```python
from build123d import *
from build123d.topology import SkipClean

# Parameters (mm, degrees)
SKETCH1_R               = 101.6
BOSS_EXTRUDE1_DEPTH     = 12.7
BOSS_EXTRUDE3_DEPTH     = 177.8
FILLET3_R               = 43.18
SKETCH3_R               = 25.4
CUT_EXTRUDE1_DEPTH      = 229.600000167
CUT_EXTRUDE2_DEPTH      = 276.632670899
CUT_EXTRUDE2_DEPTH_BACK = 276.632670899
SKETCH4_R               = 14.2875
CUT_EXTRUDE3_DEPTH      = 276.6326709
CUT_EXTRUDE3_DEPTH_BACK = 276.6326709
FILLET4_R               = 22.86
SKETCH7_W               = 43.18
SKETCH7_H               = 10
BOSS_EXTRUDE4_DEPTH     = 42.418
BOSS_EXTRUDE5_DEPTH     = 43.18
FILLET5_R               = 17.78


with BuildPart() as part:
    # Sketch1 → Boss-Extrude1 (new body)
    with BuildSketch(Plane(origin=(0, 0, 0), x_dir=(1, 0, 0), z_dir=(0, 1, 0))):
        with Locations(Location((0, 0, 0), (0, 0, 270))):
            Circle(SKETCH1_R)
    extrude(amount=BOSS_EXTRUDE1_DEPTH)

    # Sketch2 → Boss-Extrude3 (add)
    with SkipClean():  # the faces are left unmerged after this step: merging them gives an invalid solid
        with BuildSketch(Plane(origin=(0, 12.7, 0), x_dir=(1, 0, 0), z_dir=(0, 1, 0))):
            with BuildLine():
                Line((-69.749231612, -34.987681034), (-95.385649738, -34.987681034))
                ThreePointArc((-95.385649738, -34.987681034), (-101.6, 0), (-95.385649738, 34.987681034))
                Line((-95.385649738, 34.987681034), (-69.749231612, 34.987681034))
                Line((-69.749231612, 34.987681034), (-69.749231612, -34.987681034))
            make_face()
            with BuildLine():
                Line((69.749231612, 34.987681034), (95.385649738, 34.987681034))
                ThreePointArc((95.385649738, 34.987681034), (101.6, 0), (95.385649738, -34.987681034))
                Line((95.385649738, -34.987681034), (69.749231612, -34.987681034))
                Line((69.749231612, -34.987681034), (69.749231612, 34.987681034))
            make_face()
        extrude(amount=BOSS_EXTRUDE3_DEPTH)

    # Fillet3
    # the kernel refuses this fillet: 43.18 mm, written as the material it adds along each edge
    with BuildSketch(Plane(origin=(-203.335649738, 12.7, -34.987681034), x_dir=(0, 0, -1), z_dir=(1, 0, 0))) as fillet3_piece_1_section:
        with BuildLine():
            CenterArc((FILLET3_R, FILLET3_R), FILLET3_R, 180, 90)
            Line((0, FILLET3_R), (0, 0))
            Line((0, 0), (FILLET3_R, 0))
        make_face()
    fillet3_piece_1 = extrude(amount=133.586418126, mode=Mode.PRIVATE)
    fillet3_piece_1 = fillet3_piece_1 & Plane(origin=(0, 23.799745308, 0), x_dir=(0, 0, 1), z_dir=(0, -1, 0)) * Cylinder(101.6, 440, mode=Mode.PRIVATE)
    add(fillet3_piece_1)
    with BuildSketch(Plane(origin=(203.335649738, 12.7, 34.987681034), x_dir=(0, 0, 1), z_dir=(-1, 0, 0))) as fillet3_piece_2_section:
        with BuildLine():
            CenterArc((FILLET3_R, FILLET3_R), FILLET3_R, 180, 90)
            Line((0, FILLET3_R), (0, 0))
            Line((0, 0), (FILLET3_R, 0))
        make_face()
    fillet3_piece_2 = extrude(amount=133.586418126, mode=Mode.PRIVATE)
    fillet3_piece_2 = fillet3_piece_2 & Plane(origin=(0, 23.799745308, 0), x_dir=(0, 0, 1), z_dir=(0, -1, 0)) * Cylinder(101.6, 440, mode=Mode.PRIVATE)
    add(fillet3_piece_2)
    with BuildSketch(Plane(origin=(69.749231612, 12.7, -34.987681034), x_dir=(0, 0, -1), z_dir=(1, 0, 0))) as fillet3_piece_3_section:
        with BuildLine():
            CenterArc((FILLET3_R, FILLET3_R), FILLET3_R, 180, 90)
            Line((0, FILLET3_R), (0, 0))
            Line((0, 0), (FILLET3_R, 0))
        make_face()
    fillet3_piece_3 = extrude(amount=133.586418126, mode=Mode.PRIVATE)
    fillet3_piece_3 = fillet3_piece_3 & Plane(origin=(0, 23.79973444, 0), x_dir=(0, 0, 1), z_dir=(0, -1, 0)) * Cylinder(101.6, 440, mode=Mode.PRIVATE)
    add(fillet3_piece_3)
    with BuildSketch(Plane(origin=(-69.749231612, 12.7, 34.987681034), x_dir=(0, 0, 1), z_dir=(-1, 0, 0))) as fillet3_piece_4_section:
        with BuildLine():
            CenterArc((FILLET3_R, FILLET3_R), FILLET3_R, 180, 90)
            Line((0, FILLET3_R), (0, 0))
            Line((0, 0), (FILLET3_R, 0))
        make_face()
    fillet3_piece_4 = extrude(amount=133.586418126, mode=Mode.PRIVATE)
    fillet3_piece_4 = fillet3_piece_4 & Plane(origin=(0, 23.79973444, 0), x_dir=(0, 0, 1), z_dir=(0, -1, 0)) * Cylinder(101.6, 440, mode=Mode.PRIVATE)
    add(fillet3_piece_4)

    # Sketch3 → Cut-Extrude1 (cut, through all)
    with BuildSketch(Plane(origin=(0, 12.7, 0), x_dir=(1, 0, 0), z_dir=(0, 1, 0))):
        with Locations(Location((0, 0, 0), (0, 0, 270))):
            Circle(SKETCH3_R)
    extrude(amount=-CUT_EXTRUDE1_DEPTH, mode=Mode.SUBTRACT)

    # Sketch4 → Cut-Extrude2 (cut, two sides: drawn at the far end of the back side and taken through both)
    with BuildSketch(Plane.ZY.offset(-69.749231612).offset(-CUT_EXTRUDE2_DEPTH_BACK)):
        with Locations((0, 165.1)):
            Circle(SKETCH4_R)
    extrude(amount=CUT_EXTRUDE2_DEPTH + CUT_EXTRUDE2_DEPTH_BACK, mode=Mode.SUBTRACT)

    # Sketch5 → Cut-Extrude3 (cut, two sides: drawn at the far end of the back side and taken through both)
    with BuildSketch(Plane.ZY.offset(-69.749231612).offset(-CUT_EXTRUDE3_DEPTH_BACK)):
        with BuildLine():
            Line((34.987681034, 160.366849855), (34.987681034, 209.992755937))
            Line((34.987681034, 209.992755937), (-34.987681034, 209.992755937))
            Line((-34.987681034, 209.992755937), (-34.987681034, 160.366849855))
            ThreePointArc((-34.987681034, 160.366849855), (0, 195.354530889), (34.987681034, 160.366849855))
        make_face()
    extrude(amount=CUT_EXTRUDE3_DEPTH + CUT_EXTRUDE3_DEPTH_BACK, mode=Mode.SUBTRACT)

    # Fillet4
    fillet4_edges = [part.edges().sort_by_distance(p)[0] for p in [
        (-84.890685507, 190.5, -17.780075547),
        (-84.890685507, 190.5, 17.780075547),
        (84.890685507, 190.5, -17.780075547),
        (84.890685507, 190.5, 17.780075547),
    ]]
    fillet(fillet4_edges, radius=FILLET4_R)

    # Sketch7 → Boss-Extrude4 (add)
    with BuildSketch(Plane(origin=(0, 12.7, 0), x_dir=(1, 0, 0), z_dir=(0, 1, 0))):
        with Locations((-48.159231612, 26.209)):
            Rectangle(SKETCH7_W, SKETCH7_H)
        with Locations((-48.159231612, -26.209)):
            Rectangle(SKETCH7_W, SKETCH7_H)
    extrude(amount=BOSS_EXTRUDE4_DEPTH)

    # Sketch8 → Boss-Extrude5 (add)
    with BuildSketch(Plane(origin=(-69.749231612, 0, 0), x_dir=(0, 0, -1), z_dir=(1, 0, 0))):
        Polygon((-21.209, 17.78), (-21.209, 12.7), (-16.891, 12.7), align=None)
        Polygon((16.891, 12.7), (21.209, 17.78), (21.209, 12.7), align=None)
    extrude(amount=BOSS_EXTRUDE5_DEPTH)

    # Fillet5
    fillet5_edges = [part.edges().sort_by_distance(p)[0] for p in [
        (-48.159231612, 12.7, -31.209),
        (-48.159231612, 12.7, 31.209),
    ]]
    fillet(fillet5_edges, radius=FILLET5_R)


solid = part.part
```
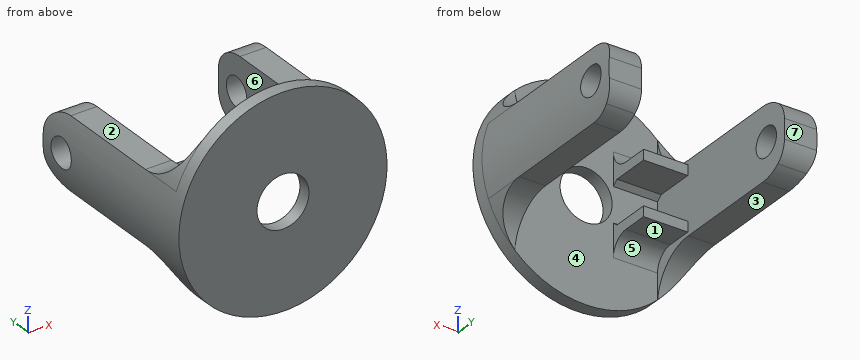
Build history of the part. All positions in model axes, mm. Face numbers are marked on the shaded views. A direction names the side the tool comes from. Round coordinates to 2 decimals unless told otherwise and drop trailing zeros. Loops run counter-clockwise (first coordinate to the right, second up) from the corner with the lowest first, then second, coordinate; pieces in that order, holes last.
Item 1: Saw through at C-C (y = 165.1). List the corners of the cut face in (x, z), then the cut area to 3 significant figures.
Item 2: Saw through at B-B (z = 0). List the corners of the cut face in (x, y).
Item 3: Saw through at A-A (x = 0). List the corners of the cut face in (y, z), then the cut area to 3 significant figures.
Item 4: Pin check, flat tips, straight feed: P1, Ø8, axis at x = 75, z = 29, coming from the +Y side; P2, Ø6, axis at y = 23.5, z = -5, coming from the +X side; P3, Ø9.5, axis at y = 31, z = -40, coming from the +X side. Stop position of each tip, or through.
Item 5: Which spindle directions (+Z, -Z, +X, -X, +Y, -Y) get a long thin tool onto all of the face, cutting with end or side? Do the marked faces 1, 2, 3 and 4. Say none if no direction does.
Item 6: Two-plate mould, pull along X, no slides. Class the marked faces 5, 6 and 7: released by +X, released by -X, zero draft, split by the parting line, or undercut.
Item 7: Saw through at D-D (y = 37). List the corners of the cut face in (x, z).
Item 8: Drill centre lines: line 1 along X through (y, z) = (10.25, 0); line 2 along Y through (x, z) = (-91, 0); line 3 along Y through (x, z) = (23, -27.5). Where is each one in solid material? Low to high.
Worked answers:
1. outline: (-100.59, -14.29) arc R101.6 ccw to (-95.5, -34.67) - (-69.75, -34.67) - (-69.75, -14.29) - close; (-100.59, 14.29) - (-69.75, 14.29) - (-69.75, 34.67) - (-95.5, 34.67) arc R101.6 ccw to start; (69.75, -34.67) - (95.5, -34.67) arc R101.6 ccw to (100.59, -14.29) - (69.75, -14.29) - close; (69.75, 14.29) - (100.59, 14.29) arc R101.6 ccw to (95.5, 34.67) - (69.75, 34.67) - close
1. area: 2,340 mm2
2. outline: (-101.6, 0) - (-25.4, 0) - (-25.4, 12.7) - (-69.75, 12.7) - (-69.75, 150.81) - (-101.6, 150.81) - close; (-101.6, 179.39) - (-69.75, 179.39) - (-69.75, 190.5) - (-101.6, 190.5) - close; (25.4, 0) - (101.6, 0) - (101.6, 150.81) - (69.75, 150.81) - (69.75, 12.7) - (25.4, 12.7) - close; (69.75, 179.39) - (101.6, 179.39) - (101.6, 190.5) - (69.75, 190.5) - close
3. outline: (0, -101.6) - (12.7, -101.6) - (12.7, -25.4) - (0, -25.4) - close; (0, 25.4) - (12.7, 25.4) - (12.7, 101.6) - (0, 101.6) - close
3. area: 1,940 mm2
4. P1: stops at y = 184.63
4. P2: stops at x = 101.58
4. P3: stops at x = 95.29
5. face 1: -Z, +Y
5. face 2: +Z, +X, -X, +Y
5. face 3: -Z, +X, -X, +Y
5. face 4: +Y
6. face 5: undercut
6. face 6: undercut
6. face 7: zero draft
7. outline: (-93.68, -39.33) - (-69.75, -39.33) - (-69.75, -31.21) - (-26.57, -31.21) - (-26.57, -21.21) - (-69.75, -21.21) - (-69.75, 21.21) - (-26.57, 21.21) - (-26.57, 31.21) - (-69.75, 31.21) - (-69.75, 39.33) - (-93.68, 39.33) arc R101.6 ccw to start; (69.75, -39.33) - (93.68, -39.33) arc R101.6 ccw to (93.68, 39.33) - (69.75, 39.33) - close
8. line 1: x = -101.6 to -25.4, 25.4 to 101.6
8. line 2: y = 0 to 150.81, 179.39 to 190.5
8. line 3: y = 0 to 12.7
